Can you work these out from the model? Positions are in its coordinate system, mm. Face numbers are marked on the shaded views. A direction names the side the tool comes from. Round coordinates to 2 decimals unless told otherwise and drop trailing zeros. Loops run counter-clockwise (first coordinate to the right, second up) from the corner with the lowest first, then second, coordinate; pieces in that order, holes last. Notation, with made-up numbers: (28.25, 82) -> (44.25, 82) arc R21 cw to (44.25, 102) -> close; hole circle Ø2 at (27.5, 79.5). An arc over 180 degrees is marked (long way). Answer as a JSON object with one key per item and string values.
```python
from build123d import *

# Parameters (mm, degrees)
EXTRUDE_1_DEPTH = 60
EXTRUDE_2_DEPTH = 10


with BuildPart() as part:
    # 草图1 → 凸台-拉伸1 (new body)
    with BuildSketch(Plane.XY):
        Polygon((-19.732146976, -1.598220465), (-11.732146976, -1.598220465), (-11.732146976, 3.401779535), (-15.732146976, 3.401779535), (-15.732146976, 8.401779535), (16.267853024, 8.401779535), (16.267853024, 3.401779535), (12.267853024, 3.401779535), (12.267853024, -1.598220465), (20.267853024, -1.598220465), (20.267853024, 22.401779535), (-19.732146976, 22.401779535), align=None)
    extrude(amount=EXTRUDE_1_DEPTH)

    # 草图2 → 凸台-拉伸2 (add)
    with BuildSketch(Plane.XZ.offset(1.598220465)):
        with BuildLine():
            Line((-29.732146976, 51.166010489), (-19.732146976, 51.166010489))
            Line((-19.732146976, 51.166010489), (-19.732146976, 8.833989511))
            Line((-19.732146976, 8.833989511), (-29.732146976, 8.833989511))
            ThreePointArc((-29.732146976, 8.833989511), (-55.52111794, -1.949954349), (-79.945012394, 11.645554037))
            ThreePointArc((-79.945012394, 11.645554037), (-78.962709962, 17.216467959), (-73.391796039, 16.234165528))
            ThreePointArc((-73.391796039, 16.234165528), (-29.732146976, 30), (-73.391796039, 43.765834472))
            ThreePointArc((-73.391796039, 43.765834472), (-78.962709962, 42.783532041), (-79.945012394, 48.354445963))
            ThreePointArc((-79.945012394, 48.354445963), (-55.52111794, 61.949954349), (-29.732146976, 51.166010489))
        make_face()
    extrude(amount=-EXTRUDE_2_DEPTH)


solid = part.part
```
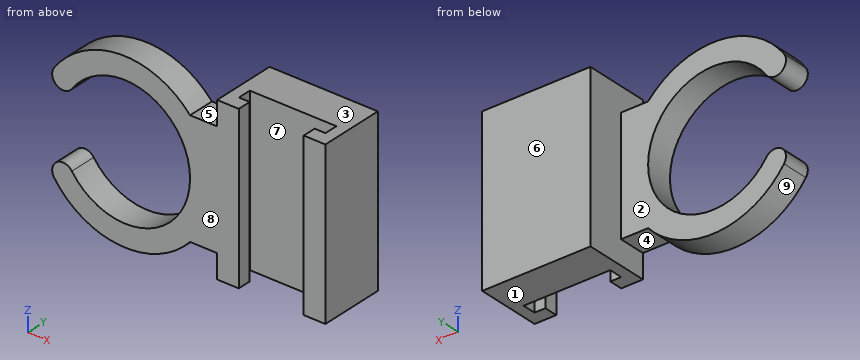
Q1. I'm going to push flat-ended pins straight in: pin 1 (11 mm diameter, centred on x = -26, y = 5.5, fed in from +Z); pin 2 (5.5 mm diameter, centred on y = 0, z = 25, fed in from -X); pin 3 (16 mm diameter, centred on x = -7, z = 21, fed in from -Y); pin 4 (4 mm diameter, centred on y = 5, z = 40.5, fed in from -X). Where does each tip first touch, or does it pass through?
Determined:
{"pin 1": "z = 53.02", "pin 2": "x = -31.02", "pin 3": "y = -1.6", "pin 4": "x = -78.49"}
Q2. I want a section at B-B, the plane z = 30. Write out the boundary of the cut face in (x, y).
Determined:
{"outline": "(-29.73, -1.6) -> (-11.73, -1.6) -> (-11.73, 3.4) -> (-15.73, 3.4) -> (-15.73, 8.4) -> (16.27, 8.4) -> (16.27, 3.4) -> (12.27, 3.4) -> (12.27, -1.6) -> (20.27, -1.6) -> (20.27, 22.4) -> (-19.73, 22.4) -> (-19.73, 8.4) -> (-29.73, 8.4) -> close"}
Q3. I want a section at A-A, the plane x = -39. Write out the boundary of the cut face in (y, z), then the cut area to 3 significant figures.
Determined:
{"outline": "(-1.6, 1.59) -> (8.4, 1.59) -> (8.4, 11.05) -> (-1.6, 11.05) -> close; (-1.6, 48.95) -> (8.4, 48.95) -> (8.4, 58.41) -> (-1.6, 58.41) -> close", "area": "189 mm²"}
Q4. If I drill on L1, parallel to X at y = 4.25, z = 30; L2, parallel to Y at x = -23.5, z = 17; L3, parallel to X at y = 1.75, z = 44, over which ranges is the centre line in solid material (lowest first)? Write a range as [from, to].
Determined:
{"L1": "[-29.73, -15.73], [16.27, 20.27]", "L2": "[-1.6, 8.4]", "L3": "[-80.1, -73.23], [-34.24, -11.73], [12.27, 20.27]"}
Q5. On a 3-axis mill with a long thin cutter (end or side, diameter ignored), from which of +Z, -Z, +X, -X, +Y, -Y can I reach the whole of each face in a straight line? I mean the marked faces 1, 2, 3, 4 and 5. Say none if no direction works.
Determined:
{"face 1": "-Z, +X, +Y, -Y", "face 2": "+Z, -Z, -X, +Y", "face 3": "+Z, +X, +Y, -Y", "face 4": "-Z, +Y, -Y", "face 5": "+Z, +Y, -Y"}
Q6. We'd pull the mould along Y, two halves only. Please class the marked faces 6, 7, 8 and 9: pulls with the +Y half, pulls with the -Y half, needs draft (parallel to the pull), parting line crosses it, or undercut.
Determined:
{"face 6": "pulls with the +Y half", "face 7": "undercut", "face 8": "pulls with the -Y half", "face 9": "needs draft"}
Q7. I want a section at C-C, the plane y = 0.25. Write out the boundary of the cut face in (x, z), then the cut area to 3 significant figures.
Determined:
{"outline": "(-79.95, 11.65) arc R32 ccw to (-29.73, 8.83) -> (-19.73, 8.83) -> (-19.73, 0) -> (-11.73, 0) -> (-11.73, 60) -> (-19.73, 60) -> (-19.73, 51.17) -> (-29.73, 51.17) arc R32 ccw to (-79.95, 48.35) arc R4 ccw to (-73.39, 43.77) arc R24 cw (long way) to (-73.39, 16.23) arc R4 ccw to start; (12.27, 0) -> (20.27, 0) -> (20.27, 60) -> (12.27, 60) -> close", "area": "2,340 mm²"}
Q8. I want a section at D-D, the plane y = 20. Write out the boundary of the cut face in (x, z), then the cut area to 3 significant figures.
Determined:
{"outline": "(-19.73, 0) -> (20.27, 0) -> (20.27, 60) -> (-19.73, 60) -> close", "area": "2,400 mm²"}
